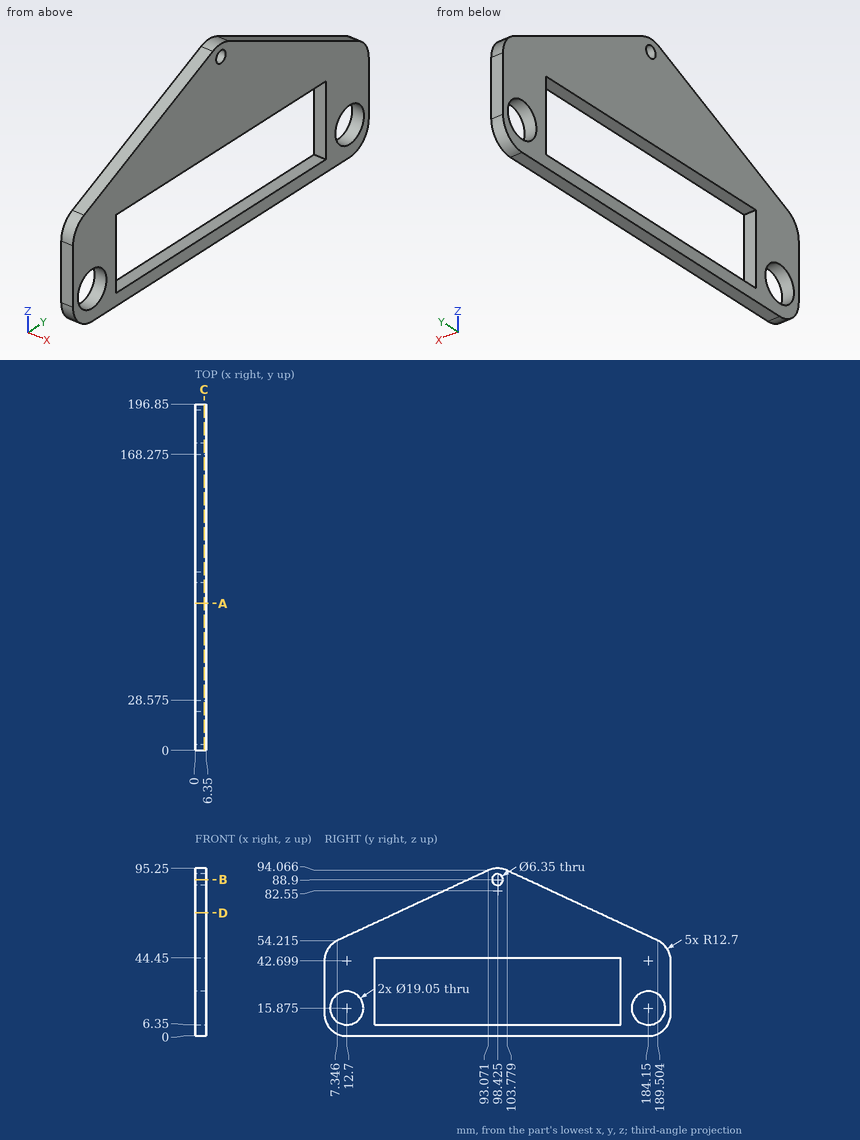
Answer from the drawing. Dimensions are ordinates in mm from the lowest x, y and z of the part. Give positions to 0.01 mm unless a question says otherwise; leave off trailing zeros. Order: outer loops, then holes, each group sorted by start corner. A loop starts at its lowest first (then second) coordinate and runs counter-clockwise, first axis right, second up.
Item 1: Given pin 1 Ø17 at (y, z) = (12.7, 15.875) entering from -X; pin 2 Ø3 at (x, y) = (2.5, 103) entering from +Z, each flat-ended and moving along its own axis, determine where each tip first touches the part or whether it passes through.
From the geometry:
pin 1: passes through
pin 2: stops at z = 94.87
Item 2: The part is cut by section D-D, the plane z = 70. Give the vertices of the cut face in (x, y).
From the geometry:
outline: (0, 41.3) - (6.35, 41.3) - (6.35, 155.55) - (0, 155.55) - close
Item 3: Find the intervals of material crossed by probe 1 along Y at (x, z) = (1.75, 10) (1 decimal); probe 2 along Y at (x, z) = (5.5, 43.5) (1 decimal); probe 3 along Z at (x, y) = (0.5, 133.5), in increasing order.
From the geometry:
probe 1: y = 0.3 to 5.2, 20.2 to 28.6, 168.3 to 176.7, 191.6 to 196.6
probe 2: y = 0 to 28.6, 168.3 to 196.8
probe 3: z = 0 to 6.35, 44.45 to 80.25
Item 4: The part is cut by section C-C, the plane x = 5. Count the separate pieces of the cut face and the enclosed holes in it, and give its area (3 significant figures).
From the geometry:
separate pieces: 1
enclosed holes: 4
area: 8,480 mm2
Item 5: The part is cut by section B-B, the plane z = 88.9. Give the vertices of the cut face in (x, y).
From the geometry:
outline: (0, 81.96) - (6.35, 81.96) - (6.35, 95.25) - (0, 95.25) - close; (0, 101.6) - (6.35, 101.6) - (6.35, 114.89) - (0, 114.89) - close
Item 6: The part is cut by section A-A, the plane y = 83.5. Give the vertices of the cut face in (x, z).
From the geometry:
outline: (0, 0) - (6.35, 0) - (6.35, 6.35) - (0, 6.35) - close; (0, 44.45) - (6.35, 44.45) - (6.35, 89.62) - (0, 89.62) - close
